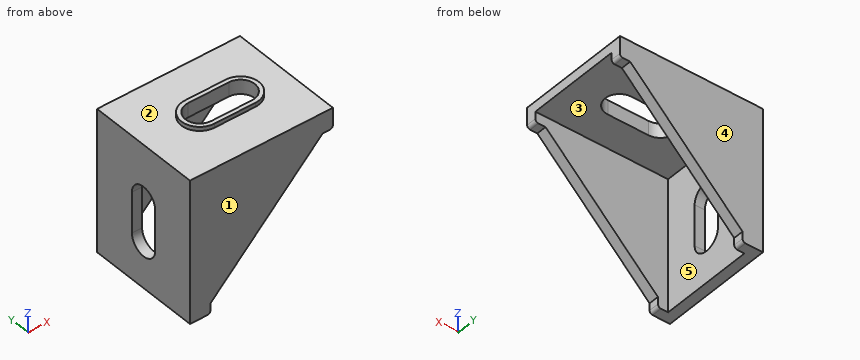
```python
from build123d import *

# Parameters (mm, degrees)
BOSS_EXTRUDE1_DEPTH = 28
BOSS_EXTRUDE2_DEPTH = 2.5
BOSS_EXTRUDE3_START = -25.5
BOSS_EXTRUDE3_DEPTH = 2.5
CUT_EXTRUDE1_DEPTH  = 2.5
CUT_EXTRUDE2_DEPTH  = 2.5
BOSS_EXTRUDE4_DEPTH = 1


with BuildPart() as part:
    # Sketch1 → Boss-Extrude1 (new body)
    with BuildSketch(Plane(origin=(0, 0, 0), x_dir=(1, 0, 0), z_dir=(0, 1, 0))):
        Polygon((0, 0), (0, 35), (2.5, 35), (2.5, 2.5), (35, 2.5), (35, 0), align=None)
    extrude(amount=BOSS_EXTRUDE1_DEPTH)

    # Sketch2 → Boss-Extrude2 (add)
    with BuildSketch(Plane(origin=(0, 28, 0), x_dir=(1, 0, 0), z_dir=(0, 1, 0))):
        with BuildLine():
            Line((2.5, 35), (4.25, 35))
            ThreePointArc((4.25, 35), (4.780330086, 34.780330086), (5, 34.25))
            Line((5, 34.25), (5, 32.5))
            Line((5, 32.5), (32.5, 5))
            Line((32.5, 5), (34.25, 5))
            ThreePointArc((34.25, 5), (34.780330086, 4.780330086), (35, 4.25))
            Line((35, 4.25), (35, 2.5))
            Line((35, 2.5), (2.5, 2.5))
            Line((2.5, 2.5), (2.5, 35))
        make_face()
    extrude(amount=-BOSS_EXTRUDE2_DEPTH)

    # Sketch2<2> → Boss-Extrude3 (add)
    with BuildSketch(Plane(origin=(0, 28, 0), x_dir=(1, 0, 0), z_dir=(0, 1, 0)).offset(BOSS_EXTRUDE3_START)):
        with BuildLine():
            Line((2.5, 35), (4.25, 35))
            ThreePointArc((4.25, 35), (4.780330086, 34.780330086), (5, 34.25))
            Line((5, 34.25), (5, 32.5))
            Line((5, 32.5), (32.5, 5))
            Line((32.5, 5), (34.25, 5))
            ThreePointArc((34.25, 5), (34.780330086, 4.780330086), (35, 4.25))
            Line((35, 4.25), (35, 2.5))
            Line((35, 2.5), (2.5, 2.5))
            Line((2.5, 2.5), (2.5, 35))
        make_face()
    extrude(amount=-BOSS_EXTRUDE3_DEPTH)

    # Sketch3 → Cut-Extrude1 (cut)
    with BuildSketch(Plane(origin=(0, 0, -2.5), x_dir=(-1, 0, 0), z_dir=(0, 0, -1))):
        with BuildLine():
            Line((-23.75, 17.5), (-13.75, 17.5))
            ThreePointArc((-13.75, 17.5), (-10.25, 14), (-13.75, 10.5))
            Line((-13.75, 10.5), (-23.75, 10.5))
            ThreePointArc((-23.75, 10.5), (-27.25, 14), (-23.75, 17.5))
        make_face()
    extrude(amount=-CUT_EXTRUDE1_DEPTH, mode=Mode.SUBTRACT)

    # Sketch4 → Cut-Extrude2 (cut)
    with BuildSketch(Plane(origin=(2.5, 0, 0), x_dir=(0, 0, -1), z_dir=(1, 0, 0))):
        with BuildLine():
            Line((13.75, 17.5), (23.75, 17.5))
            ThreePointArc((23.75, 17.5), (27.25, 14), (23.75, 10.5))
            Line((23.75, 10.5), (13.75, 10.5))
            ThreePointArc((13.75, 10.5), (10.25, 14), (13.75, 17.5))
        make_face()
    extrude(amount=-CUT_EXTRUDE2_DEPTH, mode=Mode.SUBTRACT)

    # Sketch5 → Boss-Extrude4 (add)
    with BuildSketch(Plane.XY):
        with BuildLine():
            Line((13.75, 18.5), (23.75, 18.5))
            ThreePointArc((23.75, 18.5), (28.25, 14), (23.75, 9.5))
            Line((23.75, 9.5), (13.75, 9.5))
            ThreePointArc((13.75, 9.5), (9.25, 14), (13.75, 18.5))
        make_face()
        with BuildLine():
            Line((13.75, 17.5), (23.75, 17.5))
            ThreePointArc((23.75, 17.5), (27.25, 14), (23.75, 10.5))
            Line((23.75, 10.5), (13.75, 10.5))
            ThreePointArc((13.75, 10.5), (10.25, 14), (13.75, 17.5))
        make_face(mode=Mode.SUBTRACT)
    extrude(amount=BOSS_EXTRUDE4_DEPTH)


solid = part.part
```
Source: CAD feature listing. Evaluate the final solid. Frame: model axes, mm. Face numbers are marked on the shaded views. A direction names the side the tool comes from. Give positions to 0.01 mm unless a question says otherwise; leave off trailing zeros. Loops run counter-clockwise (first coordinate to the right, second up) from the corner with the lowest first, then second, coordinate; pieces in that order, holes last. Notation, with made-up numbers: M 39,-35 L 87,-35 A15 cw 87,-8 Z; hole C 8,34.5 d10. An arc over 180 degrees is marked long. Put each result on its own line as item: value.
Q1. Section C-C (y = 16.25). Return the cut outline in (x, z).
Response values:
outline: M 0,-35 L 2.5,-35 L 2.5,-26.43 L 0,-26.43 Z; M 0,-11.07 L 2.5,-11.07 L 2.5,-2.5 L 11.07,-2.5 L 11.07,1 L 9.85,1 L 9.85,0 L 0,0 Z; M 26.43,-2.5 L 35,-2.5 L 35,0 L 27.65,0 L 27.65,1 L 26.43,1 Z
Q2. Line query: probe 1 along Y at (x, z) = (6, -6); probe 2 along Y at (x, z) = (23, -1.5); probe 3 along X at (y, z) = (7.75, -7.5). Output: solid intervals per line, ascending. Write a range as [from, to].
Response values:
probe 1: y = [0, 2.5], [25.5, 28]
probe 2: y = [0, 10.5], [17.5, 28]
probe 3: x = [0, 2.5]
Q3. Section A-A (x = 19.5). Return the cut outline in (y, z), and give its area (3 significant figures).
Response values:
outline: M 0,-18 L 2.5,-18 L 2.5,-2.5 L 10.5,-2.5 L 10.5,1 L 9.5,1 L 9.5,0 L 0,0 Z; M 17.5,-2.5 L 25.5,-2.5 L 25.5,-18 L 28,-18 L 28,0 L 18.5,0 L 18.5,1 L 17.5,1 Z
area: 132 mm²
Q4. Reachability of the marked faces 4 and 5 from +Z, -Z, +X, -X, +Y, -Y: full face, straight path, thin tool, end or side. Return the list, or none.
Response values:
face 4: +Z, -Z, +X, -X, +Y
face 5: -Z, +X
Q5. Section D-D (x = 8). Return the cut outline in (y, z), and give its area (3 significant figures).
Response values:
outline: M 0,-29.5 L 2.5,-29.5 L 2.5,-2.5 L 25.5,-2.5 L 25.5,-29.5 L 28,-29.5 L 28,0 L 0,0 Z
area: 205 mm²
Q6. Pin query (flat end, axial travel): P1, Ø14, axis at x = 15.5, y = 14.5, coming from the +Z side; P2, Ø4, axis at y = 14, z = -11, coming from the +X side; P3, Ø5, axis at x = 15, y = 11.5, coming from the -Z side; P4, Ø1.9, axis at x = 33, y = 1.5, coming from the -Z side. Return the tip coordinate at first contact, or that it passes through.
Response values:
P1: stops at z = 1
P2: stops at x = 2.5
P3: stops at z = -2.5
P4: stops at z = -5.45
Q7. Section B-B (z = -16.5). Return the cut outline in (x, y).
Response values:
outline: M 0,0 L 21,0 L 21,2.5 L 2.5,2.5 L 2.5,10.5 L 0,10.5 Z; M 0,17.5 L 2.5,17.5 L 2.5,25.5 L 21,25.5 L 21,28 L 0,28 Z
Q8. Mould query, pull axis Y, two halves, no side actions, for the marked faces 1, 2 and 3. Classes: released by +Y, released by -Y, zero draft, split by the parting line, or undercut.
Response values:
face 1: released by -Y
face 2: zero draft
face 3: undercut
